Source: CAD feature listing. Evaluate the final solid. Frame: model axes, mm. A direction names the side the tool comes from. Give positions to 0.01 mm unless a question says otherwise; leave off trailing zeros. Loops run counter-clockwise (first coordinate to the right, second up) from the corner with the lowest first, then second, coordinate; pieces in that order, holes last. Notation, with made-up numbers: M -22.75,18.25 L 32.25,18.25 A22 cw 32.25,27.25 Z; hole C -4,79.25 d2. An arc over 180 degrees is marked long. Answer in a Markdown table with one row per item.
```python
from build123d import *

# Parameters (mm, degrees)
F0_R     = 3.925
F1_DEPTH = 5
F0_R_2   = 5
F2_DEPTH = 2
F3_R     = 1


with BuildPart() as f1:
    # F0 (on Top) → F1 (new body, symmetric)
    with BuildSketch(Plane.XY):
        Circle(F0_R)
    extrude(amount=F1_DEPTH, both=True)

    # F0 (on Top) → F2 (join, symmetric)
    with BuildSketch(Plane.XY):
        Circle(F0_R_2)
        Circle(F0_R, mode=Mode.SUBTRACT)
    extrude(amount=F2_DEPTH, both=True)

    # F3
    f3_edges = [f1.edges().sort_by_distance(p)[0] for p in [
        (-5, 0, 2),
        (-5, 0, -2),
    ]]
    fillet(f3_edges, radius=F3_R)


solid = f1.part
```
1) Section C-C, the plane z = -3.25. Return loops of the section in (x, y) (3 decimals).
Reply:
| item | result |
|---|---|
| outline | C 0,0 d7.85 |
2) Material intervals for L1, parallel to X at y = -2.5, z = 1; L2, parallel to Z at x = -3.25, y = -3.25; L3, parallel to Y at x = 0.25, z = 1, sorted ascending.
Reply:
| item | result |
|---|---|
| L1 | x = -4.33 to 4.33 |
| L2 | z = -1.8 to 1.8 |
| L3 | y = -4.99 to 4.99 |
3) Pin query (flat end, axial travel): pin 1 Ø4 at (x, z) = (3.5, 1.5) entering from -Y; pin 2 Ø1.5 at (x, z) = (2.5, -2.5) entering from -Y. Return the tip coordinate at first contact, or that it passes through.
Reply:
| item | result |
|---|---|
| pin 1 | stops at y = -4.75 |
| pin 2 | stops at y = -4.02 |
4) Section A-A, the plane x = 0. Return loops of the section in (y, z) (3 decimals).
Reply:
| item | result |
|---|---|
| outline | M -5,-1 A1 ccw -4,-2 L -3.925,-2 L -3.925,-5 L 3.925,-5 L 3.925,-2 L 4,-2 A1 ccw 5,-1 L 5,1 A1 ccw 4,2 L 3.925,2 L 3.925,5 L -3.925,5 L -3.925,2 L -4,2 A1 ccw -5,1 Z |
5) Set-up query: faces 1 (the flat face through (0, 0, 5)), 2 (the cylindrical face through (-2.893, 2.653, 3.521)), 3 (the cylindrical face through (-2.893, 2.653, -3.479)). Return all of +Z, -Z, +X, -X, +Y, -Y with unobstructed straight access to the full face (end or side cutting, diameter ignored); none if empty.
Reply:
| item | result |
|---|---|
| face 1 | +Z, +X, -X, +Y, -Y |
| face 2 | +Z |
| face 3 | -Z |
